from build123d import *

# Parameters (mm, degrees)
SKETCH1_W           = 19.05
SKETCH1_H           = 111.125
BOSS_EXTRUDE1_DEPTH = 1.5875
SKETCH2_W           = 14.2875
SKETCH2_H           = 6.35
CUT_EXTRUDE1_DEPTH  = 4.175


with BuildPart() as part:
    # Sketch1 → Boss-Extrude1 (new body, symmetric)
    with BuildSketch(Plane(origin=(0, 0, 0), x_dir=(0, 0, -1), z_dir=(1, 0, 0))):
        Rectangle(SKETCH1_W, SKETCH1_H)
    extrude(amount=BOSS_EXTRUDE1_DEPTH, both=True)

    # Sketch2 → Cut-Extrude1 (cut, through all)
    with BuildSketch(Plane(origin=(1.5875, 0, 0), x_dir=(0, 0, -1), z_dir=(1, 0, 0))):
        with Locations((-2.38125, 52.3875)):
            Rectangle(SKETCH2_W, SKETCH2_H)
        with Locations((-2.38125, 17.4625)):
            Rectangle(SKETCH2_W, SKETCH2_H)
    extrude(amount=-CUT_EXTRUDE1_DEPTH, mode=Mode.SUBTRACT)


solid = part.part
The model under review builds one solid part; all positions refer to its coordinate system, in mm. A direction names the side the tool comes from. Coordinates: 2 decimals unless noted, no trailing zeros. Loops run counter-clockwise (first coordinate to the right, second up) from the corner with the lowest first, then second, coordinate; pieces in that order, holes last. Notation, with made-up numbers: (48.25, 7) -> (55.25, 7) arc R32 ccw to (55.25, 39) -> close; hole circle Ø7 at (1, 79.25). An arc over 180 degrees is marked (long way). Use a Markdown table: item, result. Add a question column.
1. Add section A-A on z = 3. Write out the cut boundary in (x, y).
2. Draft analysis for pull direction Y (two halves, no side actions). For faces 1 (the face through (0, 49.213, 2)), 2 (the face through (0, 14.287, 2)), 3 (the face through (-1.588, 1, 0)), state which applies: pulls with the +Y half, pulls with the -Y half, needs draft (parallel to the pull), parting line crosses it, or undercut.
3. Machinability: for faces 4 (the face through (0, 20.638, 2)), 5 (the face through (0, -55.562, 0)), 6 (the face through (0, 52, -4.762)), which of the approach directions +Z, -Z, +X, -X, +Y, -Y give a long, thin tool a straight path to every point of the face, cutting with its end or side? Answer none if there is none.
4. Add section B-B on x = 0.85. Write out the cut boundary in (y, z) (1 decimal).
5. Clearance check with flat-ended pins moving along their axes: pin 1 Ø1 at (x, z) = (0.5, 2) entering from +Y; pin 2 Ø1 at (x, y) = (0, 54) entering from +Z. State where each tip first meets the part, or that it passes through.
6. To check wall thickness, follow line 1 (Y direction, x = 0.85, z = 1.75); line 2 (Z direction, x = 0.15, y = 18) (1 decimal). State the ranges of each line that lie inside material, in increasing order.
Returned:
| question | item | result |
|---|---|---|
| 1 | outline | (-1.59, -55.56) -> (1.59, -55.56) -> (1.59, 14.29) -> (-1.59, 14.29) -> close; (-1.59, 20.64) -> (1.59, 20.64) -> (1.59, 49.21) -> (-1.59, 49.21) -> close |
| 2 | face 1 | pulls with the +Y half |
| 2 | face 2 | undercut |
| 2 | face 3 | needs draft |
| 3 | face 4 | +Z, +X, -X |
| 3 | face 5 | +Z, -Z, +X, -X, -Y |
| 3 | face 6 | +Z, +X, -X, +Y |
| 4 | outline | (-55.6, -9.5) -> (55.6, -9.5) -> (55.6, -4.8) -> (49.2, -4.8) -> (49.2, 9.5) -> (20.6, 9.5) -> (20.6, -4.8) -> (14.3, -4.8) -> (14.3, 9.5) -> (-55.6, 9.5) -> close |
| 5 | pin 1 | stops at y = 49.21 |
| 5 | pin 2 | stops at z = -4.76 |
| 6 | line 1 | y = -55.56 to 14.29, 20.64 to 49.21 |
| 6 | line 2 | z = -9.5 to -4.8 |
